Geometry check sheet. Reference: the model listing, model coordinates, mm. Face numbers are marked on the shaded views. A direction names the side the tool comes from. Round coordinates to 2 decimals unless told otherwise and drop trailing zeros. Write each loop counter-clockwise with the first axis right and the second up, starting at its lowest first coordinate (ties: lowest second). Pieces come first, ordered by that corner, then holes. Notation, with made-up numbers: (88, 55.25) - (98, 55.25) arc R8 ccw to (98, 63.25) - close; hole circle Ø5 at (50.25, 14). An arc over 180 degrees is marked (long way). Return JSON: item names as keys, results as strings. Group by question number.
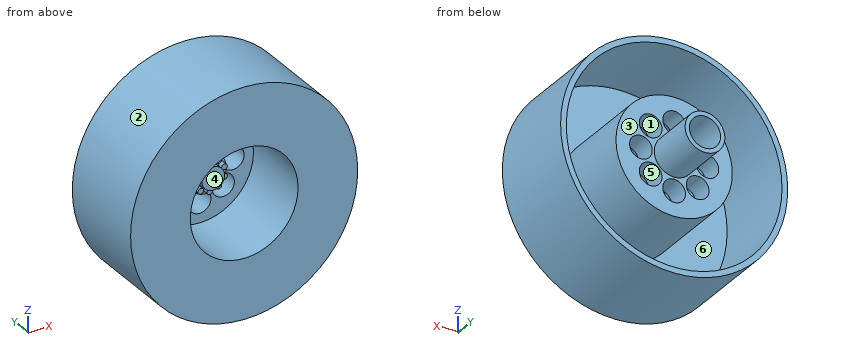
from build123d import *

# Parameters (mm, degrees)
F0_R      = 20
F1_DEPTH  = 17
F2_R      = 9.5
F3_DEPTH  = 13
F4_R      = 2
F5_DEPTH  = 4
F6_R      = 3.5
F7_DEPTH  = 2
F8_R      = 2
F9_DEPTH  = 2
F10_R     = 0.5
F11_DEPTH = 1
F12_R     = 3.5
F13_DEPTH = 9
F14_R     = 2.75
F15_DEPTH = 9
F16_R     = 19
F16_R_2   = 9.5
F17_DEPTH = 16
F18_R     = 10.25
F18_R_2   = 9.5
F19_DEPTH = 17


# Not quite as in the source:
# - a feature names something its author has since deleted; it is built from what else it names


with BuildPart() as f1:
    # F0 (on Front) → F1 (new body)
    with BuildSketch(Plane.XZ):
        Circle(F0_R)
    extrude(amount=F1_DEPTH)

    # F2 (on face) → F3 (cut)
    with BuildSketch(Plane.XZ.offset(17)):
        Circle(F2_R)
    extrude(amount=-F3_DEPTH, mode=Mode.SUBTRACT)

    # F4 (on face) → F5 (cut)
    with BuildSketch(Plane.XZ.offset(4)):
        with Locations((-4.1401582032, 4.1401582032)):
            Circle(F4_R)
        with Locations((0, 5.8550678814)):
            Circle(F4_R)
        with Locations((4.1401582032, 4.1401582032)):
            Circle(F4_R)
        with Locations((5.8550678814, 0)):
            Circle(F4_R)
        with Locations((4.1401582032, -4.1401582032)):
            Circle(F4_R)
        with Locations((0, -5.8550678814)):
            Circle(F4_R)
        with Locations((-4.1401582032, -4.1401582032)):
            Circle(F4_R)
        with Locations((-5.8550678814, 0)):
            Circle(F4_R)
    extrude(amount=-F5_DEPTH, mode=Mode.SUBTRACT)

    # F6 (on face) → F7 (join)
    with BuildSketch(Plane.XZ.offset(4)):
        Circle(F6_R)
    extrude(amount=F7_DEPTH)

    # F8 (on face) → F9 (join)
    with BuildSketch(Plane.XZ.offset(6)):
        Circle(F8_R)
    extrude(amount=F9_DEPTH)

    # F10 (on face) → F11 (join)
    with BuildSketch(Plane.XZ.offset(6)):
        with Locations((0, 2.7124709893)):
            Circle(F10_R)
        with Locations((1.5943504448, 2.1944351271)):
            Circle(F10_R)
        with Locations((2.5797132096, 0.8381996324)):
            Circle(F10_R)
        with Locations((2.5797132096, -0.8381996324)):
            Circle(F10_R)
        with Locations((1.5943504448, -2.1944351271)):
            Circle(F10_R)
        with Locations((0, -2.7124709893)):
            Circle(F10_R)
        with Locations((-1.5943504448, -2.1944351271)):
            Circle(F10_R)
        with Locations((-2.5797132096, -0.8381996324)):
            Circle(F10_R)
        with Locations((-2.5797132096, 0.8381996324)):
            Circle(F10_R)
        with Locations((-1.5943504448, 2.1944351271)):
            Circle(F10_R)
    extrude(amount=F11_DEPTH)

    # F12 (on face) → F13 (join)
    with BuildSketch(Plane(origin=(0, 0, 0), x_dir=(-1, 0, 0), z_dir=(0, 1, 0))):
        Circle(F12_R)
    extrude(amount=F13_DEPTH)

    # F14 (on face) → F15 (cut)
    with BuildSketch(Plane(origin=(0, 9, 0), x_dir=(-1, 0, 0), z_dir=(0, 1, 0))):
        Circle(F14_R)
    extrude(amount=-F15_DEPTH, mode=Mode.SUBTRACT)

    # F16 (on face) → F17 (cut)
    with BuildSketch(Plane(origin=(0, 0, 0), x_dir=(-1, 0, 0), z_dir=(0, 1, 0))):
        Circle(F16_R)
        Circle(F16_R_2, mode=Mode.SUBTRACT)
    extrude(amount=-F17_DEPTH, mode=Mode.SUBTRACT)

    # F18 (on face) → F19 (join)
    with BuildSketch(Plane.XZ.offset(17)):
        Circle(F18_R)
        Circle(F18_R_2, mode=Mode.SUBTRACT)
    extrude(amount=-F19_DEPTH)


solid = f1.part
1. Section check D-D (z = -15). Enter the section's corners in (x, y).
2. Material ranges on line 1 along Z through (x, y) = (0, -13.75); line 2 along Z through (x, y) = (0, -3); line 3 along Z through (x, y) = (-8, -8.75), recorded low to high.
3. Section check A-A (y = -4.5). Enter the section's corners in (x, z), and give its area (3 significant figures).
4. Depth check by flat-ended pin: pin 1 Ø4.5 at (x, z) = (-5.86, 0) entering from +Y; pin 2 Ø0.8 at (x, z) = (1.5, 2.5) entering from -Y; pin 3 Ø8 at (x, z) = (13.5, -5.5) entering from +Y. Enter the tip coordinate at first touch or a pass-through.
5. Section check B-B (y = -12). Enter the section's corners in (x, z), and give its area (3 significant figures).
6. Mould release check, pull along X, two halves, no side actions. Record for the marked faces 1, 2 and 3: pulls with the +X half, pulls with the -X half, needs draft (parallel to the pull), parting line crosses it, or undercut.
7. Section check C-C (x = 0). State how many separate pieces and enclosed holes the cut face has, and give its area (4 significant figures).
8. Tool access check on the marked faces 4, 5 and 6. Record the directions out of +Z, -Z, +X, -X, +Y, -Y that give a thin tool (end or side, any length) a straight path to the whole face; none if there is none.
Result sheet:
{
 "1": {"outline": "(-13.23, -17) - (13.23, -17) - (13.23, 0) - (11.66, 0) - (11.66, -16) - (-11.66, -16) - (-11.66, 0) - (-13.23, 0) - close"},
 "2": {"line 1": "z = -20 to -19, -10.25 to -9.5, 9.5 to 10.25, 19 to 20", "line 2": "z = -20 to -19, -10.25 to -7.86, -3.86 to 3.86, 7.86 to 10.25, 19 to 20", "line 3": "z = -18.33 to -17.23, -6.41 to -5.12, 5.12 to 6.41, 17.23 to 18.33"},
 "3": {"outline": "circle Ø40 at (0, 0); circle Ø20.5 at (0, 0); circle Ø7 at (0, 0); hole circle Ø38 at (0, 0); hole circle Ø19 at (0, 0)", "area": "208 mm²"},
 "4": {"pin 1": "stops at y = 0", "pin 2": "stops at y = -7", "pin 3": "stops at y = -16"},
 "5": {"outline": "circle Ø40 at (0, 0); circle Ø20.5 at (0, 0); hole circle Ø38 at (0, 0); hole circle Ø19 at (0, 0)", "area": "169 mm²"},
 "6": {"face 1": "undercut", "face 2": "parting line crosses it", "face 3": "needs draft"},
 "7": {"separate pieces": "3", "enclosed holes": "0", "area": "158.5 mm²"},
 "8": {"face 4": "-Y", "face 5": "+Y, -Y", "face 6": "+Y"}
}
